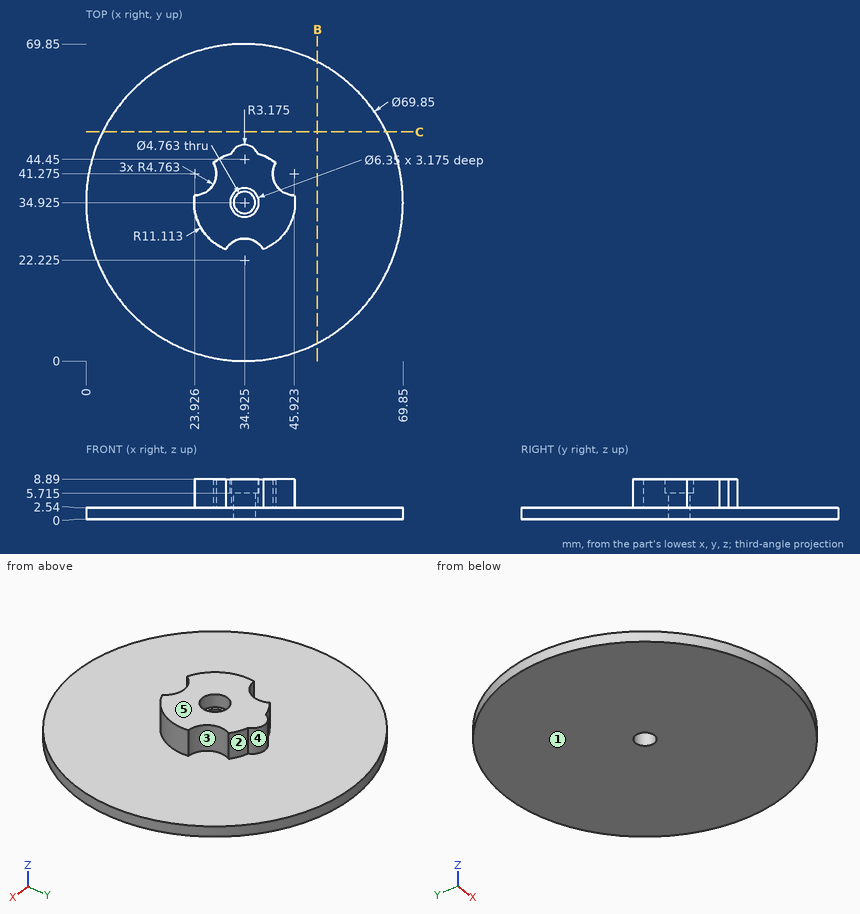
The figure shows three views and two pictorial views of one solid part (mm, origin at its lowest corner). Answer the questions. A direction names the side the tool comes from. Give positions to 0.01 mm unless a question says otherwise; leave off trailing zeros. Order: outer loops, then holes, each group sorted by start corner. A loop starts at its lowest first (then second) coordinate and runs counter-clockwise, first axis right, second up. Notation, with made-up numbers: (49, -19) -> (55, -19) arc R18 cw to (55, -2) -> close; hole circle Ø10 at (29.5, 81). An arc over 180 degrees is marked (long way). Write each question's results on one line, items separated by ' | '.
Q1. Each of these flat-tipped pins is pushed along its axis until it touches: P1, Ø7, axis at x = 33.5, y = 35.5, coming from the +Z side; P2, Ø5, axis at x = 34.925, y = 34.925, coming from the +Z side (1 decimal); P3, Ø4.5, axis at x = 34.925, y = 34.925, coming from the -Z side; P4, Ø1, axis at x = 45.5, z = 7, coming from the +Y side. Where does it stop, or does it pass through?
Checked values:
P1: stops at z = 8.89 | P2: stops at z = 5.7 | P3: passes through | P4: stops at y = 36.6
Q2. Determine the mould class of the marked faces 1, 2 and 3 for opening direction Y: pulls with the +Y half, pulls with the -Y half, needs draft (parallel to the pull), parting line crosses it, or undercut.
Checked values:
face 1: needs draft | face 2: pulls with the +Y half | face 3: undercut
Q3. Straight lines are drawn through the part: probe 1 along Z at (x, y) = (21, 24.5); probe 2 along Y at (x, z) = (33.5, 4) (1 decimal); probe 3 along Y at (x, z) = (37, 2) (1 decimal). For each, find the intervals that lie inside material, in ascending order. Write a range as from..to.
Checked values:
probe 1: z = 0..2.54 | probe 2: y = 26.8..33, 36.8..47.3 | probe 3: y = 0.1..33.8, 36.1..69.8
Q4. The part is cut by section B-B, the plane x = 51. Give the vertices of the cut face in (y, z).
Checked values:
outline: (3.92, 0) -> (65.93, 0) -> (65.93, 2.54) -> (3.92, 2.54) -> close
Q5. Which of the six approach directions +Z, -Z, +X, -X, +Y, -Y give full straight-line access (tool end or side, diameter ignored) to the marked faces 4 and 5?
Checked values:
face 4: +Z, +Y | face 5: +Z, +X, -X, +Y, -Y
Q6. The part is cut by section C-C, the plane y = 50.5. Give the vertices of the cut face in (x, z) (1 decimal).
Checked values:
outline: (3.7, 0) -> (66.2, 0) -> (66.2, 2.5) -> (3.7, 2.5) -> close
